Autodesk Inventor part; units mm, degrees
ref_plane "YZ Plane" through (0, 0, 0) normal (1, 0, 0) x (0, 1, 0)
ref_plane "XZ Plane" through (0, 0, 0) normal (0, 1, 0) x (-1, 0, 0)
ref_plane "XY Plane" through (0, 0, 0) normal (0, 0, 1) x (1, 0, 0)
sketch "スケッチ2" plane through (0, 0, 0) normal (0, 1, 0) x (-1, 0, 0)
  line L0 (0, 0) -> (-170, 0)
  line L1 (-170, 0) -> (-170, -233)
  line L2 (-170, -233) -> (0, -233)
  line L3 (0, -233) -> (0, 0)
  dimension "d0" = 170
  dimension "d1" = 233
extrude "押し出し1" add sketch "スケッチ2" along normal blind 34
fillet "フィレット1" radius 10 4 edges at (170, 17, 0) (0, 17, 0) (170, 17, -233) (0, 17, -233)
fillet "フィレット2" radius 3 16 edges at (167.0711, 34, -2.9289) (170, 34, -116.5) (167.0711, 34, -230.0711) (85, 34, -233) (2.9289, 34, -230.0711) (0, 34, -116.5) (2.9289, 34, -2.9289) (85, 34, 0) (167.0711, 0, -230.0711) (85, 0, -233) (2.9289, 0, -230.0711) (0, 0, -116.5) (2.9289, 0, -2.9289) (85, 0, 0) (167.0711, 0, -2.9289) (170, 0, -116.5)
sketch "スケッチ3" plane through (0, 34, 0) normal (0, 1, 0) x (1, 0, 0)
  line L0 (10, 10) -> (13, 10)
  line L1 (13, 10) -> (13, 25)
  line L2 (13, 25) -> (10, 25)
  line L3 (10, 25) -> (10, 10)
  line L4 (0, 223) -> (0, 10)
  line L5 (10, 0) -> (160, 0)
  line L6 (157, 10) -> (160, 10)
  line L7 (160, 10) -> (160, 25)
  line L8 (160, 25) -> (157, 25)
  line L9 (157, 25) -> (157, 10)
  line L10 (170, 10) -> (170, 223)
  arc A0 (170, 223) -> (160, 233) centre (160, 223) ccw
  line L11 (160, 223) -> (157, 223)
  line L12 (157, 223) -> (157, 208)
  line L13 (157, 208) -> (160, 208)
  line L14 (160, 208) -> (160, 223)
  arc A1 (10, 233) -> (0, 223) centre (10, 223) ccw
  line L15 (10, 223) -> (13, 223)
  line L16 (13, 223) -> (13, 208)
  line L17 (13, 208) -> (10, 208)
  line L18 (10, 208) -> (10, 223)
  point P0 (0, 0)
  dimension "d6" = 3
  dimension "d7" = 15
  dimension "d8" = 10
  dimension "d9" = 10
  dimension "d10" = 3
  dimension "d11" = 15
  dimension "d12" = 10
  dimension "d13" = 10
  dimension "d14" = 3
  dimension "d15" = 15
  dimension "d16" = 3
  dimension "d17" = 15
extrude "押し出し2" add sketch "スケッチ3" along normal blind 3
properties part number "box" material "ガラス"
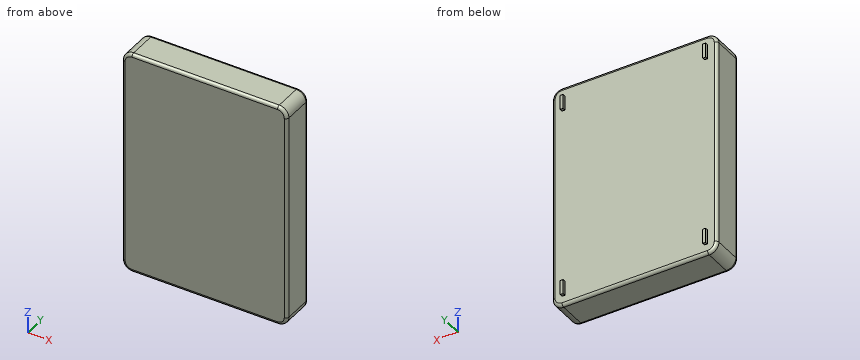
Build history of the part. All positions in model axes, mm. Round coordinates to 2 decimals unless told otherwise and drop trailing zeros. Write each loop counter-clockwise with the first axis right and the second up, starting at its lowest first coordinate (ties: lowest second). Pieces come first, ordered by that corner, then holes. Notation, with made-up numbers: (41.25, 17) - (72.25, 17) arc R28 ccw to (72.25, 39) - close; hole circle Ø5 at (68, 48). An arc over 180 degrees is marked (long way). Answer as CSV lines item,"result".
Q1. Drop flat-ended pins along their axis: pin 1 (0.9 mm diameter, centred on x = 12, y = 35.5, fed in from +Z); pin 2 (1.5 mm diameter, centred on x = 158.5, y = 36, fed in from -Z); pin 3 (3.5 mm diameter, centred on y = 36, z = -215.5, fed in from -X); pin 4 (10 mm diameter, centred on x = 87.5, z = -151.5, fed in from -Y). Give the stop position or say it passes through.
Report:
pin 1,"stops at z = -10"
pin 2,"stops at z = -223"
pin 3,"stops at x = 10"
pin 4,"stops at y = 0"
Q2. Drill centre lines: probe 1 along X at (y, z) = (35.5, -219); probe 2 along Y at (x, z) = (144.5, -35); probe 3 along Z at (x, y) = (160.5, 21.5). Where is each one in solid material? Low to high. Write a range as [from, to].
Report:
probe 1,"x = [10, 13], [157, 160]"
probe 2,"y = [0, 34]"
probe 3,"z = [-232.99, -0.01]"
Q3. Cut at C-C (z = -219). Write the cut outline in (x, y).
Report:
outline,"(0, 3) arc R3 ccw to (3, 0) - (167, 0) arc R3 ccw to (170, 3) - (170, 31) arc R3 ccw to (167, 34) - (160, 34) - (160, 37) - (157, 37) - (157, 34) - (13, 34) - (13, 37) - (10, 37) - (10, 34) - (3, 34) arc R3 ccw to (0, 31) - close"
Q4. Cut at A-A (z = -180.5). Write the cut outline in (x, y), and give its area (3 significant figures).
Report:
outline,"(0, 3) arc R3 ccw to (3, 0) - (167, 0) arc R3 ccw to (170, 3) - (170, 31) arc R3 ccw to (167, 34) - (3, 34) arc R3 ccw to (0, 31) - close"
area,"5,770 mm^2"
Q5. Cut at B-B (x = 37). Write the cut outline in (y, z).
Report:
outline,"(0, -230) arc R3 ccw to (3, -233) - (31, -233) arc R3 ccw to (34, -230) - (34, -3) arc R3 ccw to (31, 0) - (3, 0) arc R3 ccw to (0, -3) - close"
